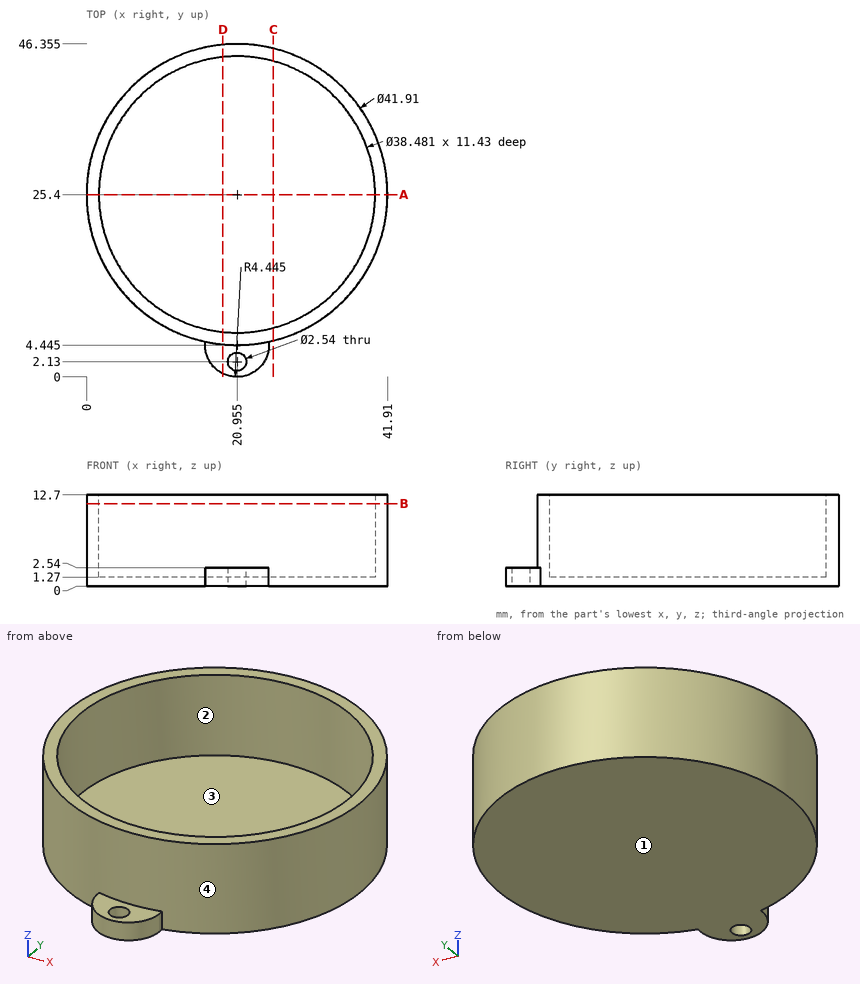
The drawing under review shows one solid part. Ordinate dimensions are in mm from its lowest x, y, z. Coordinates: 2 decimals unless noted, no trailing zeros. Write each loop counter-clockwise with the first axis right and the second up, starting at its lowest first coordinate (ties: lowest second). Pieces come first, ordered by that corner, then holes. Notation, with made-up numbers: (-38, 89) - (-3, 89) arc R18 ccw to (-3, 105) - close; hole circle Ø1 at (15.5, 35). An arc over 180 degrees is marked (long way). Put each result on its own line as item: value.
1. Add section B-B, the plane z = 11.5. Give the boundary of the cut face in (x, y) (1 decimal).
Values found:
outline: circle Ø41.9 at (21, 25.4); hole circle Ø38.5 at (21, 25.4)
2. Mouldability with a two-part tool opening along Y and no side actions: class the marked faces 1, 2, 3 and 4 as released by +Y, released by -Y, zero draft, split by the parting line, or undercut.
Values found:
face 1: zero draft
face 2: undercut
face 3: undercut
face 4: split by the parting line
3. For pin 1 (6 mm diameter, centred on y = 11.5, z = 1.5, fed in from +X); pin 2 (2 mm diameter, centred on y = 26.5, z = 9.5, fed in from +X); pin 3 (6 mm diameter, centred on x = 15.5, z = 5, fed in from +Y); pin 4 (1.5 mm diameter, centred on x = 19.5, y = 2, fed in from +Z), all flat-tipped, find the tip position at first contact; note any pin that passes through.
Values found:
pin 1: x = 38.85
pin 2: x = 41.91
pin 3: y = 46.21
pin 4: z = 2.54
4. Add section D-D, the plane x = 19. Give the boundary of the cut face in (y, z).
Values found:
outline: (0.45, 0) - (46.26, 0) - (46.26, 12.7) - (44.54, 12.7) - (44.54, 1.27) - (6.26, 1.27) - (6.26, 12.7) - (4.54, 12.7) - (4.54, 2.54) - (0.45, 2.54) - close
5. Add section A-A, the plane y = 25.4. Give the boundary of the cut face in (x, z) (1 decimal).
Values found:
outline: (0, 0) - (41.9, 0) - (41.9, 12.7) - (40.2, 12.7) - (40.2, 1.3) - (1.7, 1.3) - (1.7, 12.7) - (0, 12.7) - close
6. Wall thickness on probe 1 along X at (y, z) = (25.4, 7) (1 decimal); probe 2 along Y at (x, z) = (21, 3.5) (1 decimal); probe 3 along Z at (x, y) = (20, 39.5): over which ranges is each line inside the solid? List them lowest first.
Values found:
probe 1: 0 to 1.7, 40.2 to 41.9
probe 2: 4.4 to 6.2, 44.6 to 46.4
probe 3: 0 to 1.27
7. Add section C-C, the plane x = 26. Give the boundary of the cut face in (y, z).
Values found:
outline: (5.06, 0) - (45.74, 0) - (45.74, 12.7) - (43.97, 12.7) - (43.97, 1.27) - (6.83, 1.27) - (6.83, 12.7) - (5.06, 12.7) - close
